```python
from build123d import *

# Parameters (mm, degrees)
SKETCH_1_W          = 20
SKETCH_1_H          = 55.6
EXTRUDE_1_DEPTH     = 3
SKETCH_2_W          = 4
SKETCH_2_H          = 5
EXTRUDE_2_DEPTH     = 3
SKETCH_3_W          = 6.666666666
SKETCH_3_H          = 2.2
SKETCH_3_R          = 1.5
SKETCH_3_R_2        = 3
SKETCH_3_H_2        = 1.6
CUT_EXTRUDE_1_DEPTH = 10


with BuildPart() as part:
    # 草图1 → 凸台-拉伸1 (new body)
    with BuildSketch(Plane(origin=(0, 0, 0), x_dir=(1, 0, 0), z_dir=(0, 1, 0))):
        with Locations((-10, -27.8)):
            Rectangle(SKETCH_1_W, SKETCH_1_H)
    extrude(amount=EXTRUDE_1_DEPTH)

    # 草图2 → 凸台-拉伸2 (add)
    with BuildSketch(Plane(origin=(0, 3, 0), x_dir=(1, 0, 0), z_dir=(0, 1, 0))):
        with Locations((-14, 2.5)):
            Rectangle(SKETCH_2_W, SKETCH_2_H)
        with Locations((-6, 2.5)):
            Rectangle(SKETCH_2_W, SKETCH_2_H)
        with Locations((-14, -58.1)):
            Rectangle(SKETCH_2_W, SKETCH_2_H)
        with Locations((-6, -58.1)):
            Rectangle(SKETCH_2_W, SKETCH_2_H)
    extrude(amount=-EXTRUDE_2_DEPTH)

    # 草图3 → 切除-拉伸1 (cut)
    with BuildSketch(Plane(origin=(0, 3, 0), x_dir=(1, 0, 0), z_dir=(0, 1, 0))):
        with Locations((-10, -52.3)):
            Rectangle(SKETCH_3_W, SKETCH_3_H)
        with Locations(Location((-5.050252532, -31.849747468, 0), (0, 0, 270))):
            Circle(SKETCH_3_R)
        with Locations(Location((-10, -26.9, 0), (0, 0, 270))):
            Circle(SKETCH_3_R_2)
        with Locations((-10, -2.4)):
            Rectangle(SKETCH_3_W, SKETCH_3_H_2)
        with Locations(Location((-14.949747468, -31.849747468, 0), (0, 0, 270))):
            Circle(SKETCH_3_R)
        with Locations(Location((-14.949747468, -21.950252532, 0), (0, 0, 270))):
            Circle(SKETCH_3_R)
        with Locations(Location((-5.050252532, -21.950252532, 0), (0, 0, 270))):
            Circle(SKETCH_3_R)
    extrude(amount=-CUT_EXTRUDE_1_DEPTH, mode=Mode.SUBTRACT)


solid = part.part
```
Geometry check sheet. Reference: the model listing, model coordinates, mm. A direction names the side the tool comes from. Give positions to 0.01 mm unless a question says otherwise; leave off trailing zeros. Loops run counter-clockwise (first coordinate to the right, second up) from the corner with the lowest first, then second, coordinate; pieces in that order, holes last. Notation, with made-up numbers: M 69.5,82 L 114.5,82 A14 cw 114.5,89 Z; hole C 63.5,39.5 d6. An arc over 180 degrees is marked long. Write item = value, one per line.
(1) Gauge pin test, flat ends, axial feed: pin 1 Ø1.5 at (x, y) = (-11, 1) entering from +Z; pin 2 Ø0.9 at (y, z) = (1, 59) entering from +X. Record the tip position at first contact, or that the pin passes through.
Answer below:
pin_1 = 55.6
pin_2 = -4
(2) Release check for a two-part mould opening along Z. For faces 5 (the face through (-10, 2, 51.2)), 6 (the face through (-14, 2, 60.6)), 7 (the face through (-18, 1, 0)), 8 (the face through (-10, 2, 1.6)) record: released by +Z, released by -Z, zero draft, split by the parting line, or undercut.
Answer below:
face_5 = undercut
face_6 = released by +Z
face_7 = released by -Z
face_8 = undercut
(3) Tool access check on faces 1 (the face through (-13.333, 2, 2)), 2 (the face through (-18, 1, 55.6)), 3 (the face through (-2, 1, 55.6)), 4 (the face through (-10, 1, 0)). Record the directions out of +Z, -Z, +X, -X, +Y, -Y that give a thin tool (end or side, any length) a straight path to the whole face; none if there is none.
Answer below:
face_1 = +Y, -Y
face_2 = +Z, -X, +Y, -Y
face_3 = +Z, +X, +Y, -Y
face_4 = -Z, +Y, -Y
(4) Sectioned sample at C-C, the plane y = 0.9. State how many separate pieces and enclosed holes the cut face has, plus the area to 3 significant figures.
Answer below:
separate_pieces = 1
enclosed_holes = 7
area = 1,110 mm2
(5) Material ranges on line 1 (X direction, y = 0.5, z = 2.5); line 2 (Z direction, x = -8.5, y = 0.3); line 3 (X direction, y = 2.75, z = 31), recorded low to high. Write a range as [from, to].
Answer below:
line_1 = [-20, -13.33], [-6.67, 0]
line_2 = [0, 1.6], [3.2, 24.3], [29.5, 51.2], [53.4, 55.6]
line_3 = [-20, -16.19], [-13.71, -6.29], [-3.81, 0]
(6) Sectioned sample at B-B, the plane z = 26.9. Record the cut outline in (x, y).
Answer below:
outline = M -20,0 L -13,0 L -13,3 L -20,3 Z; M -7,0 L 0,0 L 0,3 L -7,3 Z
(7) Sectioned sample at A-A, the plane x = -10. Record the cut outline in (y, z), plus the area to 3 significant figures.
Answer below:
outline = M 0,0 L 3,0 L 3,1.6 L 0,1.6 Z; M 0,3.2 L 3,3.2 L 3,23.9 L 0,23.9 Z; M 0,29.9 L 3,29.9 L 3,51.2 L 0,51.2 Z; M 0,53.4 L 3,53.4 L 3,55.6 L 0,55.6 Z
area = 137 mm2
(8) Sectioned sample at D-D, the plane x = -19. Record the cut outline in (y, z).
Answer below:
outline = M 0,0 L 3,0 L 3,55.6 L 0,55.6 Z
